from build123d import *

# Parameters (mm, degrees)
SKETCH1_R           = 1.5
BOSS_EXTRUDE1_DEPTH = 3
FILLET1_R           = 2
BOSS_EXTRUDE2_START = 5
SKETCH2_R           = 5.1
BOSS_EXTRUDE2_DEPTH = 10
CHAMFER1_SIZE       = 2
CHAMFER2_SIZE       = 1.5


with BuildPart() as part:
    # Sketch1 → Boss-Extrude1 (new body)
    with BuildSketch(Plane.XY):
        Polygon((10, -27.5), (25, -27.5), (25, 27.5), (-5, 27.5), (-5, 20), (-25, 20), (-25, -20), (10, -20), align=None)
        with Locations((0, 22.5)):
            Circle(SKETCH1_R, mode=Mode.SUBTRACT)
        with Locations((20, 22.5)):
            Circle(SKETCH1_R, mode=Mode.SUBTRACT)
        with Locations((20, -22.5)):
            Circle(SKETCH1_R, mode=Mode.SUBTRACT)
    extrude(amount=BOSS_EXTRUDE1_DEPTH)

    # Fillet1
    fillet1_edges = [part.edges().sort_by_distance(p)[0] for p in [
        (25, -27.5, 1.5),
        (-25, -20, 1.5),
        (-25, 20, 1.5),
        (25, 27.5, 1.5),
    ]]
    fillet(fillet1_edges, radius=FILLET1_R)

    # Sketch2 → Boss-Extrude2 (add)
    # profile 1 of 2: a face of its own
    with BuildSketch(Plane(origin=(0, 0, 0), x_dir=(0, 0, -1), z_dir=(1, 0, 0)).offset(BOSS_EXTRUDE2_START)):
        with BuildLine():
            ThreePointArc((0, -29.5), (-13.656854249, -35.156854249), (-8, -21.5))
            Line((-8, -21.5), (-3, -21.5))
            Line((-3, -21.5), (-3, -11.5))
            Line((-3, -11.5), (0, -11.5))
            Line((0, -11.5), (0, -29.5))
        make_face()
        with Locations((-8, -29.5)):
            Circle(SKETCH2_R, mode=Mode.SUBTRACT)
    # profile 2 of 2: a face of its own
    with BuildSketch(Plane(origin=(0, 0, 0), x_dir=(0, 0, -1), z_dir=(1, 0, 0)).offset(BOSS_EXTRUDE2_START)):
        with BuildLine():
            Line((0, 11.5), (0, 29.5))
            ThreePointArc((0, 29.5), (-13.656854249, 35.156854249), (-8, 21.5))
            Line((-8, 21.5), (-3, 21.5))
            Line((-3, 21.5), (-3, 11.5))
            Line((-3, 11.5), (0, 11.5))
        make_face()
        with Locations((-8, 29.5)):
            Circle(SKETCH2_R, mode=Mode.SUBTRACT)
    extrude(amount=BOSS_EXTRUDE2_DEPTH)

    # Chamfer1
    chamfer1_edges = [part.edges().sort_by_distance(p)[0] for p in [
        (-5, 20, 1.5),
        (-5, 27.5, 1.5),
    ]]
    chamfer(chamfer1_edges, length=CHAMFER1_SIZE)

    # Chamfer2
    # the kernel refuses this chamfer: 1.5 mm, written as the material it adds along each edge
    with BuildSketch(Plane(origin=(15, -21.5, 3), x_dir=(-0.02749587661058678, 0, 0.9996219169112968), z_dir=(0, -1, 0))) as chamfer2_piece_1_section:
        Polygon((CHAMFER2_SIZE * 0.999621916911, -CHAMFER2_SIZE * 0.0274958766106), (-CHAMFER2_SIZE * 0.0274958766106, -CHAMFER2_SIZE * 0.999621916911), (0, 0), align=None)
    chamfer2_piece_1 = extrude(amount=6, mode=Mode.PRIVATE)
    chamfer2_piece_1 = chamfer2_piece_1 - Plane(origin=(15.512165711, -29.5, 8), x_dir=(0, 0, -1), z_dir=(-1, 0, 0)) * Cylinder(5.1, 18, mode=Mode.PRIVATE)
    add(chamfer2_piece_1)
    with BuildSketch(Plane(origin=(5, -21.5, 3), x_dir=(0, 0.9996219169112968, -0.02749587661058648), z_dir=(1, 0, 0))) as chamfer2_piece_2_section:
        Polygon((CHAMFER2_SIZE * 0.999621916911, CHAMFER2_SIZE * 0.0274958766106), (-CHAMFER2_SIZE * 0.0274958766106, CHAMFER2_SIZE * 0.999621916911), (0, 0), align=None)
    chamfer2_piece_2 = extrude(amount=10, mode=Mode.PRIVATE)
    chamfer2_piece_2 = split(chamfer2_piece_2, bisect_by=Plane(origin=(10, -20, 3.495606231), z_dir=(0, -1, 0)), keep=Keep.TOP, mode=Mode.PRIVATE)
    add(chamfer2_piece_2)
    with BuildSketch(Plane(origin=(15, 21.5, 3), x_dir=(-0.02749587661058678, 0, 0.9996219169112968), z_dir=(0, 1, 0))) as chamfer2_piece_3_section:
        Polygon((CHAMFER2_SIZE * 0.999621916911, CHAMFER2_SIZE * 0.0274958766106), (-CHAMFER2_SIZE * 0.0274958766106, CHAMFER2_SIZE * 0.999621916911), (0, 0), align=None)
    chamfer2_piece_3 = extrude(amount=6, mode=Mode.PRIVATE)
    chamfer2_piece_3 = chamfer2_piece_3 - Plane(origin=(15.512165714, 29.5, 8), x_dir=(0, 0, -1), z_dir=(-1, 0, 0)) * Cylinder(5.1, 18, mode=Mode.PRIVATE)
    add(chamfer2_piece_3)
    with BuildSketch(Plane(origin=(5, 21.5, 3), x_dir=(0.027495876610586206, 0, 0.9996219169112968), z_dir=(0, 1, 0))) as chamfer2_piece_4_section:
        Polygon((CHAMFER2_SIZE * 0.999621916911, -CHAMFER2_SIZE * 0.0274958766106), (-CHAMFER2_SIZE * 0.0274958766106, -CHAMFER2_SIZE * 0.999621916911), (0, 0), align=None)
    chamfer2_piece_4 = extrude(amount=6, mode=Mode.PRIVATE)
    chamfer2_piece_4 = chamfer2_piece_4 - Plane(origin=(4.487834286, 29.5, 8), x_dir=(0, 0, -1), z_dir=(-1, 0, 0)) * Cylinder(5.1, 18, mode=Mode.PRIVATE)
    add(chamfer2_piece_4)
    with BuildSketch(Plane(origin=(5, 21.5, 3), x_dir=(0, -0.9996219169112968, -0.02749587661058648), z_dir=(1, 0, 0))) as chamfer2_piece_5:
        Polygon((CHAMFER2_SIZE * 0.999621916911, -CHAMFER2_SIZE * 0.0274958766106), (-CHAMFER2_SIZE * 0.0274958766106, -CHAMFER2_SIZE * 0.999621916911), (0, 0), align=None)
    extrude(amount=10)
    with BuildSketch(Plane(origin=(15, -17.642475518, 3), x_dir=(-0.02749587661058678, 0, 0.9996219169112968), z_dir=(0, -1, 0))) as chamfer2_piece_6a_section:
        Polygon((CHAMFER2_SIZE * 0.999621916911, -CHAMFER2_SIZE * 0.0274958766106), (-CHAMFER2_SIZE * 0.0274958766106, -CHAMFER2_SIZE * 0.999621916911), (0, 0), align=None)
    chamfer2_piece_6a = extrude(amount=9.857524482, mode=Mode.PRIVATE)
    chamfer2_piece_6a = split(chamfer2_piece_6a, bisect_by=Plane(origin=(15.49469044, -21.5, 3.49469044), z_dir=(0, 1, 0)), keep=Keep.TOP, mode=Mode.PRIVATE)
    with BuildSketch(Plane(origin=(5, -21.5, 3), x_dir=(0, 0.9996219169112968, -0.02749587661058648), z_dir=(1, 0, 0))) as chamfer2_piece_6b_section:
        Polygon((CHAMFER2_SIZE * 0.999621916911, CHAMFER2_SIZE * 0.0274958766106), (-CHAMFER2_SIZE * 0.0274958766106, CHAMFER2_SIZE * 0.999621916911), (0, 0), align=None)
    chamfer2_piece_6b = extrude(amount=13.857524482, mode=Mode.PRIVATE)
    chamfer2_piece_6b = split(chamfer2_piece_6b, bisect_by=Plane(origin=(16.928692538, -20, 3.495574544), z_dir=(0, -1, 0)), keep=Keep.TOP, mode=Mode.PRIVATE)
    chamfer2_piece_6b = split(chamfer2_piece_6b, bisect_by=Plane(origin=(15, -21.007028814, 3.495574544), z_dir=(1, 0, 0)), keep=Keep.TOP, mode=Mode.PRIVATE)
    chamfer2_piece_6b = chamfer2_piece_6b - Plane(origin=(20, -22.5, 3.495574544), x_dir=(1, 0, 0), z_dir=(0, 0, -1)) * Cylinder(1.5, 34, mode=Mode.PRIVATE)
    chamfer2_piece_6 = chamfer2_piece_6a & chamfer2_piece_6b
    add(chamfer2_piece_6)
    with BuildSketch(Plane(origin=(15, 17.642475518, 3), x_dir=(-0.02749587661058678, 0, 0.9996219169112968), z_dir=(0, 1, 0))) as chamfer2_piece_7a_section:
        Polygon((CHAMFER2_SIZE * 0.999621916911, CHAMFER2_SIZE * 0.0274958766106), (-CHAMFER2_SIZE * 0.0274958766106, CHAMFER2_SIZE * 0.999621916911), (0, 0), align=None)
    chamfer2_piece_7a = extrude(amount=9.857524482, mode=Mode.PRIVATE)
    chamfer2_piece_7a = split(chamfer2_piece_7a, bisect_by=Plane(origin=(15.49469044, 21.5, 3.49469044), z_dir=(0, -1, 0)), keep=Keep.TOP, mode=Mode.PRIVATE)
    with BuildSketch(Plane(origin=(5, 21.5, 3), x_dir=(0, -0.9996219169112968, -0.02749587661058648), z_dir=(1, 0, 0))) as chamfer2_piece_7b_section:
        Polygon((CHAMFER2_SIZE * 0.999621916911, -CHAMFER2_SIZE * 0.0274958766106), (-CHAMFER2_SIZE * 0.0274958766106, -CHAMFER2_SIZE * 0.999621916911), (0, 0), align=None)
    chamfer2_piece_7b = extrude(amount=13.857524482, mode=Mode.PRIVATE)
    chamfer2_piece_7b = split(chamfer2_piece_7b, bisect_by=Plane(origin=(15, 21.005289845, 3.494658773), z_dir=(1, 0, 0)), keep=Keep.TOP, mode=Mode.PRIVATE)
    chamfer2_piece_7b = chamfer2_piece_7b - Plane(origin=(20, 22.5, 3.494658773), x_dir=(1, 0, 0), z_dir=(0, 0, -1)) * Cylinder(1.5, 34, mode=Mode.PRIVATE)
    chamfer2_piece_7 = chamfer2_piece_7a & chamfer2_piece_7b
    add(chamfer2_piece_7)
    with BuildSketch(Plane(origin=(5, 17.642475518, 3), x_dir=(0.027495876610586206, 0, 0.9996219169112968), z_dir=(0, 1, 0))) as chamfer2_piece_8a_section:
        Polygon((CHAMFER2_SIZE * 0.999621916911, -CHAMFER2_SIZE * 0.0274958766106), (-CHAMFER2_SIZE * 0.0274958766106, -CHAMFER2_SIZE * 0.999621916911), (0, 0), align=None)
    chamfer2_piece_8a = extrude(amount=9.857524482, mode=Mode.PRIVATE)
    chamfer2_piece_8a = split(chamfer2_piece_8a, bisect_by=Plane(origin=(4.50530956, 21.5, 3.49469044), z_dir=(0, -1, 0)), keep=Keep.TOP, mode=Mode.PRIVATE)
    with BuildSketch(Plane(origin=(1.142475518, 21.5, 3), x_dir=(0, -0.9996219169112968, -0.02749587661058648), z_dir=(1, 0, 0))) as chamfer2_piece_8b_section:
        Polygon((CHAMFER2_SIZE * 0.999621916911, -CHAMFER2_SIZE * 0.0274958766106), (-CHAMFER2_SIZE * 0.0274958766106, -CHAMFER2_SIZE * 0.999621916911), (0, 0), align=None)
    chamfer2_piece_8b = extrude(amount=13.857524482, mode=Mode.PRIVATE)
    chamfer2_piece_8b = split(chamfer2_piece_8b, bisect_by=Plane(origin=(5, 21.005289845, 3.494658773), z_dir=(-1, 0, 0)), keep=Keep.TOP, mode=Mode.PRIVATE)
    chamfer2_piece_8b = chamfer2_piece_8b - Plane(origin=(0, 22.5, 3.494658773), x_dir=(1, 0, 0), z_dir=(0, 0, -1)) * Cylinder(1.5, 34, mode=Mode.PRIVATE)
    chamfer2_piece_8 = chamfer2_piece_8a & chamfer2_piece_8b
    add(chamfer2_piece_8)


solid = part.part
Can you work these out from the model? Positions are in its coordinate system, mm. A direction names the side the tool comes from. Round coordinates to 2 decimals unless told otherwise and drop trailing zeros. Write each loop counter-clockwise with the first axis right and the second up, starting at its lowest first coordinate (ties: lowest second). Pieces come first, ordered by that corner, then holes. Notation, with made-up numbers: (-13, 9) -> (15, 9) arc R15 ccw to (15, 14) -> close; hole circle Ø10 at (-15, -32.75). An arc over 180 degrees is marked (long way). Use one line per item in the form item = value. Start each with the question number.
Q1. Imagine slicing it at C-C (x = 10). Please give me the cut outline in (y, z), then the cut area to 3 significant figures.
Q2. We'd pull the mould along Y, two halves only. Please class faces 5 (the face through (10, -21.5, 6)), 6 (the face through (0, 0, 0)), 7 (the face through (-9, -20, 1)), 8 (the face through (10, 21.5, 6)): +Y half, -Y half, draft (parallel to the pull), parting line (faces both ways), or undercut.
Q3. I'm going to push flat-ended pins straight in: P1, Ø6, axis at x = 4, z = 1.5, coming from the +Y side; P2, Ø1, axis at x = 20, z = 1.5, coming from the +Y side; P3, Ø8, axis at y = 29.5, z = 8, coming from the +X side; P4, Ø1.1, axis at x = 10.5, z = 6, coming from the -Y side. Where does each tip first touch, or does it pass through?
Q4. Imagine slicing it at B-B (z = 9). Please give me the cut outline in (x, y), then the cut area to 3 significant figures.
Q5. If I drill on probe 1 along Y at (x, z) = (20, 0.75); probe 2 along Z at (x, y) = (10.5, -29.5); probe 3 along Y at (x, z) = (0, 0.9), over which ranges is the centre line in solid material (lowest first)? Write a range as [from, to].
Q6. Imagine slicing it at D-D (y = -22.5). Please give me the cut outline in (x, z).
Q7. Which directions (+Z, -Z, +X, -X, +Y, -Y) give clear straight access to the entire face, cutting with the end or side of a thin tool? Please do faces 1 (the face through (15, -35, 8)), 2 (the face through (5, -28.91, 2.76)), 3 (the face through (10, 21, 4)), 4 (the face through (19, -27.5, 2)).
Q8. Imagine slicing it at A-A (x = 20). Please give me the cut outline in (y, z), then the cut area to 3 significant figures.
Worked out:
q1.outline = (-29.5, 0) -> (29.5, 0) arc R8 ccw (long way) to (21.5, 8) -> (21.5, 4.5) -> (20, 3) -> (-20, 3) -> (-21.5, 4.5) -> (-21.5, 8) arc R8 ccw (long way) to start; hole circle Ø10.2 at (-29.5, 8); hole circle Ø10.2 at (29.5, 8)
q1.area = 397 mm^2
q2.face_5 = undercut
q2.face_6 = draft
q2.face_7 = -Y half
q2.face_8 = undercut
q3.P1 = 36.61
q3.P2 = 27.5
q3.P3 = through
q3.P4 = -37.37
q4.outline = (5, -37.44) -> (15, -37.44) -> (15, -34.5) -> (5, -34.5) -> close; (5, -24.5) -> (15, -24.5) -> (15, -21.56) -> (5, -21.56) -> close; (5, 21.56) -> (15, 21.56) -> (15, 24.5) -> (5, 24.5) -> close; (5, 34.5) -> (15, 34.5) -> (15, 37.44) -> (5, 37.44) -> close
q4.area = 117 mm^2
q5.probe_1 = [-27.5, -24], [-21, 21], [24, 27.5]
q5.probe_2 = [0, 2.9], [13.1, 16]
q5.probe_3 = [-20, 21], [24, 27.5]
q6.outline = (5, 0) -> (18.5, 0) -> (18.5, 3) -> (16.5, 3) -> (15, 4.5) -> (15, 11.87) -> (5, 11.87) -> close; (21.5, 0) -> (25, 0) -> (25, 3) -> (21.5, 3) -> close
q7.face_1 = +Z, +X, -Y
q7.face_2 = +Z, -Z, -X, -Y
q7.face_3 = +Z, +X, -X
q7.face_4 = +Z, -Z, +X, -Y
q8.outline = (-27.5, 0) -> (-24, 0) -> (-24, 3) -> (-27.5, 3) -> close; (-21, 0) -> (21, 0) -> (21, 3) -> (-21, 3) -> close; (24, 0) -> (27.5, 0) -> (27.5, 3) -> (24, 3) -> close
q8.area = 147 mm^2
